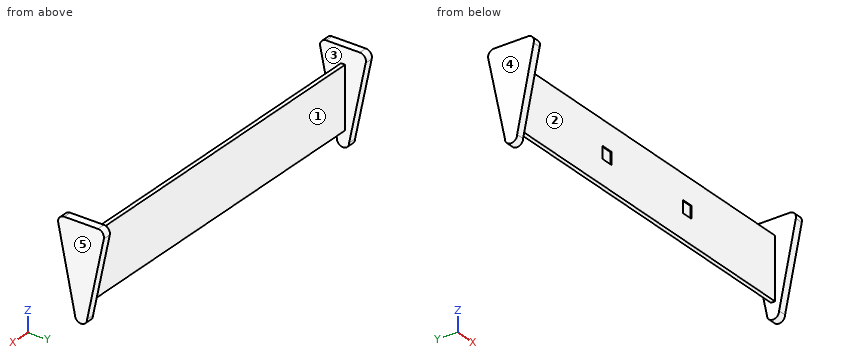
```python
from build123d import *

# Parameters (mm, degrees)
SKETCH1_W           = 90
SKETCH1_H           = 15
BOSS_EXTRUDE1_DEPTH = 0.5
BOSS_EXTRUDE2_DEPTH = 2
BOSS_EXTRUDE3_START = -2
BOSS_EXTRUDE3_DEPTH = 2
SKETCH4_W           = 3
SKETCH4_H           = 3
CUT_EXTRUDE1_DEPTH  = 0.25


with BuildPart() as part:
    # Sketch1 → Boss-Extrude1 (new, symmetric)
    with BuildSketch(Plane(origin=(0, 0, 0), x_dir=(1, 0, 0), z_dir=(0, 1, 0))):
        Rectangle(SKETCH1_W, SKETCH1_H)
    extrude(amount=BOSS_EXTRUDE1_DEPTH, both=True)

    # Sketch2 → Boss-Extrude2 (add)
    with BuildSketch(Plane(origin=(45, 0, 0), x_dir=(0, 0, -1), z_dir=(1, 0, 0))):
        with BuildLine():
            Line((-11.5, 4.142135624), (-11.5, -4.142135624))
            ThreePointArc((-11.5, -4.142135624), (-10.946118457, -5.306120102), (-9.69352018, -5.610491888))
            Line((-9.69352018, -5.610491888), (10, -1.5))
            ThreePointArc((10, -1.5), (11.5, 0), (10, 1.5))
            Line((10, 1.5), (-9.69352018, 5.610491888))
            ThreePointArc((-9.69352018, 5.610491888), (-10.946118457, 5.306120102), (-11.5, 4.142135624))
        make_face()
    extrude(amount=-BOSS_EXTRUDE2_DEPTH)

    # Sketch3 → Boss-Extrude3 (add)
    with BuildSketch(Plane.ZY.offset(45).offset(BOSS_EXTRUDE3_START)):
        with BuildLine():
            Line((-10, 1.5), (9.553557208, 5.574158261))
            ThreePointArc((9.553557208, 5.574158261), (10.888913891, 5.350370739), (11.5, 4.142135624))
            Line((11.5, 4.142135624), (11.5, -4.142135624))
            ThreePointArc((11.5, -4.142135624), (10.888913891, -5.350370739), (9.553557208, -5.574158261))
            Line((9.553557208, -5.574158261), (-10, -1.5))
            ThreePointArc((-10, -1.5), (-11.5, 0), (-10, 1.5))
        make_face()
    extrude(amount=BOSS_EXTRUDE3_DEPTH)

    # Sketch4 → Cut-Extrude1 (cut, symmetric)
    with BuildSketch(Plane.XZ.offset(0.5)):
        with Locations((13.5, 0)):
            Rectangle(SKETCH4_W, SKETCH4_H)
        with Locations((-13.5, 0)):
            Rectangle(SKETCH4_W, SKETCH4_H)
    extrude(amount=CUT_EXTRUDE1_DEPTH, both=True, mode=Mode.SUBTRACT)


solid = part.part
```
Geometry check sheet. Reference: the model listing, model coordinates, mm. Face numbers are marked on the shaded views. A direction names the side the tool comes from. Give positions to 0.01 mm unless a question says otherwise; leave off trailing zeros. Order: outer loops, then holes, each group sorted by start corner. A loop starts at its lowest first (then second) coordinate and runs counter-clockwise, first axis right, second up.
1. Release check for a two-part mould opening along X. For the marked faces 3, 4 and 5 record: pulls with the +X half, pulls with the -X half, needs draft (parallel to the pull), parting line crosses it, or undercut.
2. Thickness scan on L1, parallel to X at y = 2.5, z = 8; L2, parallel to Y at x = -34, z = -6; L3, parallel to Z at x = 16.5, y = 0.25. Record the ranges inside material, lowest first.
3. Section check C-C, the plane z = -4. Enter the section's corners in (x, y).
4. Gauge pin test, flat ends, axial feed: pin 1 Ø2 at (x, z) = (24.5, -5) entering from -Y; pin 2 Ø12 at (x, z) = (-3.5, 3.5) entering from +Y; pin 3 Ø0.8 at (x, y) = (-7, 0) entering from -Z; pin 4 Ø1 at (x, y) = (-17, -1.5) entering from -Z. Record the tip position at first contact, or that the pin passes through.
5. Access from +Z, -Z, +X, -X, +Y, -Y to the whole of each face (thin tool, end or side, straight path). Record for the marked faces 1 and 2.
6. Section check B-B, the plane x = 26. Enter the section's corners in (y, z), and give its area (3 significant figures).
7. Section check A-A, the plane y = 3.25. Enter the section's corners in (x, z), and give its area (3 significant figures).
Values follow:
1. face 3: undercut
1. face 4: pulls with the -X half
1. face 5: pulls with the +X half
2. L1: x = -45 to -43, 43 to 45
2. L2: y = -0.5 to 0.5
2. L3: z = -7.5 to 7.5
3. outline: (-45, -2.75) - (-43, -2.75) - (-43, -0.5) - (43, -0.5) - (43, -2.75) - (45, -2.75) - (45, 2.75) - (43, 2.75) - (43, 0.5) - (-43, 0.5) - (-43, 2.75) - (-45, 2.75) - close
4. pin 1: stops at y = -0.5
4. pin 2: stops at y = 0.5
4. pin 3: stops at z = -7.5
4. pin 4: passes through
5. face 1: +Z, -Z, +Y
5. face 2: +Z, -Z, -Y
6. outline: (-0.5, -7.5) - (0.5, -7.5) - (0.5, 7.5) - (-0.5, 7.5) - close
6. area: 15.0 mm2
7. outline: (-45, -1.6) - (-43, -1.6) - (-43, 11.5) - (-45, 11.5) - close; (43, -1.62) - (45, -1.62) - (45, 11.5) - (43, 11.5) - close
7. area: 52.4 mm2
